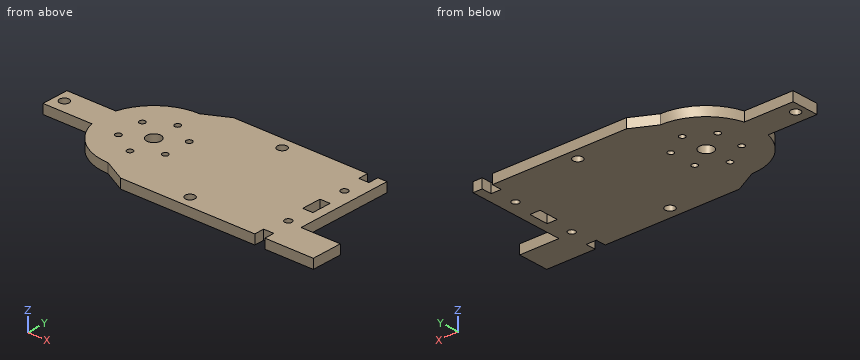
```python
from build123d import *

# Parameters (mm, degrees)
SKETCH_1_R      = 1.5
SKETCH_1_R_2    = 3
SKETCH_1_R_3    = 1.25
SKETCH_1_R_4    = 2
SKETCH_1_W      = 4.3
SKETCH_1_H      = 8.3
EXTRUDE_1_DEPTH = 4


with BuildPart() as part:
    # 草图1 → 凸台-拉伸1 (new body)
    with BuildSketch(Plane.XY):
        with BuildLine():
            Line((32.115707856, 27.15), (32.115707856, 22.85))
            Line((32.115707856, 22.85), (27.815707856, 22.85))
            Line((27.815707856, 22.85), (27.815707856, 27.15))
            Line((27.815707856, 27.15), (-29.075, 27.15))
            Line((-29.075, 27.15), (-38.998995168, 22.002009663))
            ThreePointArc((-38.998995168, 22.002009663), (-52.370174504, 17.472835843), (-60.236366221, 5.75))
            Line((-60.236366221, 5.75), (-80.958287312, 5.75))
            Line((-80.958287312, 5.75), (-80.958287312, -5.75))
            Line((-80.958287312, -5.75), (-60.236366221, -5.75))
            ThreePointArc((-60.236366221, -5.75), (-52.370174504, -17.472835843), (-38.998995168, -22.002009663))
            Line((-38.998995168, -22.002009663), (-29.075, -27.15))
            Line((-29.075, -27.15), (27.815707856, -27.15))
            Line((27.815707856, -27.15), (27.815707856, -22.85))
            Line((27.815707856, -22.85), (32.115707856, -22.85))
            Line((32.115707856, -22.85), (32.115707856, -27.15))
            Line((32.115707856, -27.15), (36.001004832, -27.15))
            Line((36.001004832, -27.15), (52.659242152, -27.15))
            Line((52.659242152, -27.15), (52.659242152, -14.15))
            Line((52.659242152, -14.15), (36.001004832, -14.15))
            Line((36.001004832, -14.15), (36.001004832, 27.15))
            Line((36.001004832, 27.15), (32.115707856, 27.15))
        make_face()
        with Locations((30.001004832, 13.5)):
            Circle(SKETCH_1_R, mode=Mode.SUBTRACT)
        with Locations(Location((30.001004832, -13.5, 0), (0, 0, 180))):
            Circle(SKETCH_1_R, mode=Mode.SUBTRACT)
        with Locations((-38.998995168, 0)):
            Circle(SKETCH_1_R_2, mode=Mode.SUBTRACT)
        with Locations((-38.998995168, -11.5)):
            Circle(SKETCH_1_R_3, mode=Mode.SUBTRACT)
        with Locations((-48.958287312, -5.75)):
            Circle(SKETCH_1_R_3, mode=Mode.SUBTRACT)
        with Locations((-48.958287312, 5.75)):
            Circle(SKETCH_1_R_3, mode=Mode.SUBTRACT)
        with Locations((-38.998995168, 11.5)):
            Circle(SKETCH_1_R_3, mode=Mode.SUBTRACT)
        with Locations((-29.039703025, 5.75)):
            Circle(SKETCH_1_R_3, mode=Mode.SUBTRACT)
        with Locations((-29.039703025, -5.75)):
            Circle(SKETCH_1_R_3, mode=Mode.SUBTRACT)
        with Locations((-4.075, -22.15)):
            Circle(SKETCH_1_R_4, mode=Mode.SUBTRACT)
        with Locations((-4.075, 22.15)):
            Circle(SKETCH_1_R_4, mode=Mode.SUBTRACT)
        with Locations((-76.958287312, 0)):
            Circle(SKETCH_1_R_4, mode=Mode.SUBTRACT)
        with Locations((30.001004832, 0)):
            Rectangle(SKETCH_1_W, SKETCH_1_H, mode=Mode.SUBTRACT)
    extrude(amount=EXTRUDE_1_DEPTH)


solid = part.part
```
Part model, mm, in its own coordinate system. Round coordinates to 2 decimals unless told otherwise and drop trailing zeros. Order: outer loops, then holes, each group sorted by start corner. A loop starts at its lowest first (then second) coordinate and runs counter-clockwise, first axis right, second up. Notation, with made-up numbers: M 57,55 L 67,55 A24 cw 67,89 Z; hole C 55,37.25 d8. An arc over 180 degrees is marked long. Put each result on its own line as item: value. Start each with the question number.
1. Drop flat-ended pins along their axis: pin 1 (2 mm diameter, centred on y = 13, z = 2, fed in from -X); pin 2 (1 mm diameter, centred on x = -48, z = 1.5, fed in from -Y); pin 3 (3 mm diameter, centred on x = -48.96, y = -5.75, fed in from -Z); pin 4 (2 mm diameter, centred on y = -14, z = 2.5, fed in from -X). Give the stop position or say it passes through.
2. Slice it at B-B on z = 3. State how many separate pieces and enclosed holes the cut face has, then the cut area to 3 significant figures.
3. Drill centre lines: probe 1 along X at (y, z) = (-23.5, 3.1); probe 2 along Y at (x, z) = (-48, 3.1); probe 3 along X at (y, z) = (2.5, 1.95). Where is each one in solid material? Low to high. Write a range as [from, to].
4. Slice it at D-D on y = 17.5. List the corners of the cut face in (x, z), then the cut area to 3 significant figures.
5. Slice it at A-A on y = 0. List the corners of the cut face in (x, z).
6. Slice it at C-C on x = -34.5. List the corners of the cut face in (y, z), then the cut area to 3 significant figures.
Findings:
1. pin 1: x = -57.44
1. pin 2: y = -20.29
1. pin 3: z = 0
1. pin 4: x = -56.75
2. separate pieces: 1
2. enclosed holes: 13
2. area: 5,050 mm2
3. probe 1: [-36.11, -5.55], [-2.6, 27.82], [32.12, 52.66]
3. probe 2: [-20.08, -6.55], [-4.95, 4.95], [6.55, 20.08]
3. probe 3: [-80.96, -40.66], [-37.34, 27.85], [32.15, 36]
4. outline: M -52.33,0 L 36,0 L 36,4 L -52.33,4 Z
4. area: 353 mm2
5. outline: M -80.96,0 L -78.96,0 L -78.96,4 L -80.96,4 Z; M -74.96,0 L -42,0 L -42,4 L -74.96,4 Z; M -36,0 L 27.85,0 L 27.85,4 L -36,4 Z; M 32.15,0 L 36,0 L 36,4 L 32.15,4 Z
6. outline: M -24.34,0 L 24.34,0 L 24.34,4 L -24.34,4 Z
6. area: 195 mm2
